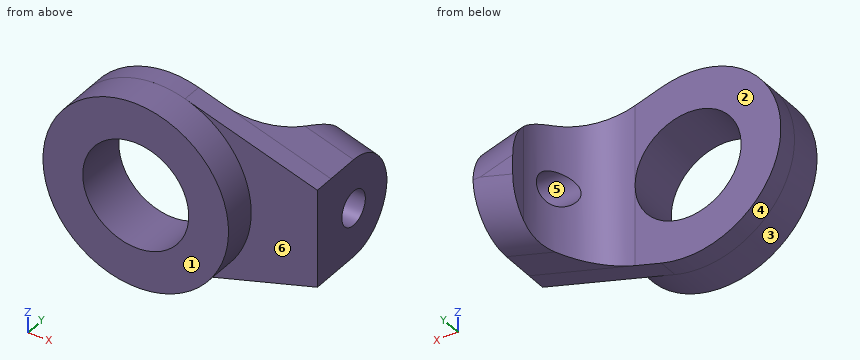
from build123d import *

# Parameters (mm, degrees)
SKETCH_1_R          = 7
EXTRUDE_1_DEPTH     = 1.5
SKETCH_3_R          = 4
CUT_EXTRUDE_2_DEPTH = 11.012492197
EXTRUDE_START       = -1.5
SKETCH_5_R          = 7
EXTRUDE_2_DEPTH     = 1.5
SKETCH_11_R         = 7
SKETCH_11_R_2       = 4
EXTRUDE_4_DEPTH     = 2.5
EXTRUDE_6_DEPTH     = 6.2
FILLET_1_R          = 5
SKETCH_12_R         = 1.3
CUT_EXTRUDE_3_DEPTH = 22.663858813
FILLET_2_R          = 3.7


with BuildPart() as part:
    # Эскиз1 → Бобышка-Вытянуть1 (new body)
    with BuildSketch(Plane(origin=(0, 0, 0), x_dir=(1, 0, 0), z_dir=(0, 1, 0))):
        with Locations(Location((0, 0, 0), (0, 0, 270))):
            Circle(SKETCH_1_R)
    extrude(amount=EXTRUDE_1_DEPTH)

    # Эскиз3 → Вырез-Вытянуть2 (cut, through all)
    with BuildSketch(Plane(origin=(0, 1.5, 0), x_dir=(1, 0, 0), z_dir=(0, 1, 0))):
        with Locations(Location((0, 0, 0), (0, 0, 270))):
            Circle(SKETCH_3_R)
    extrude(amount=-CUT_EXTRUDE_2_DEPTH, mode=Mode.SUBTRACT)

    # Эскиз5 → Бобышка-Вытянуть2 (add)
    with BuildSketch(Plane(origin=(0, 1.5, 0), x_dir=(1, 0, 0), z_dir=(0, 1, 0)).offset(EXTRUDE_START)):
        with BuildLine():
            ThreePointArc((2.017080382, 6.703746112), (-7.000630343, 0), (2.017080382, -6.703746112))
            Line((2.017080382, -6.703746112), (12, -3.7))
            Line((12, -3.7), (12, 3.7))
            Line((12, 3.7), (2.017080382, 6.703746112))
        make_face()
        Circle(SKETCH_5_R, mode=Mode.SUBTRACT)
    extrude(amount=EXTRUDE_2_DEPTH)

    # Эскиз11 → Бобышка-Вытянуть4 (add)
    with BuildSketch(Plane(origin=(0, 0, 0), x_dir=(-1, 0, 0), z_dir=(0, -1, 0))):
        with Locations(Location((0, 0, 0), (0, 0, 270))):
            Circle(SKETCH_11_R)
        with Locations(Location((0, 0, 0), (0, 0, 270))):
            Circle(SKETCH_11_R_2, mode=Mode.SUBTRACT)
    extrude(amount=EXTRUDE_4_DEPTH)

    # Эскиз13 → Бобышка-Вытянуть6 (add)
    with BuildSketch(Plane(origin=(0, 1.5, 0), x_dir=(1, 0, 0), z_dir=(0, 1, 0))):
        Polygon((9, 4.602665621), (9, 0), (9, -4.602665621), (12, -3.7), (12, 3.7), align=None)
    extrude(amount=EXTRUDE_6_DEPTH)

    # Скругление1
    fillet_1_edges = [part.edges().sort_by_distance(p)[0] for p in [
        (9, 1.5, 0),
    ]]
    fillet(fillet_1_edges, radius=FILLET_1_R)

    # Эскиз12 → Вырез-Вытянуть3 (cut, through all)
    with BuildSketch(Plane(origin=(12, 0, 0), x_dir=(0, 0, -1), z_dir=(1, 0, 0))):
        with Locations((0, 4)):
            Circle(SKETCH_12_R)
    extrude(amount=-CUT_EXTRUDE_3_DEPTH, mode=Mode.SUBTRACT)

    # Скругление2
    # the kernel refuses this fillet: 3.7 mm, written as the material it takes off along each edge
    with BuildSketch(Plane(origin=(0.142275982, 7.7, 7.267853272), x_dir=(0, -1, 0), z_dir=(0.9575917857777037, 0, -0.28812839466298473)), Plane(origin=(20.857724018, 7.7, -1.034812349), x_dir=(0, -1, 0), z_dir=(-0.9575917857777037, 0, -0.28812839466298473))) as fillet_2_piece_1:
        with BuildLine():
            CenterArc((FILLET_2_R, FILLET_2_R), FILLET_2_R, 180, 90)
            Line((0, FILLET_2_R), (0, 0))
            Line((0, 0), (FILLET_2_R, 0))
        make_face()
    extrude(amount=21.632858954, mode=Mode.SUBTRACT)


solid = part.part
Can you work these out from the model? Positions are in its coordinate system, mm. Face numbers are marked on the shaded views. A direction names the side the tool comes from. Coordinates: 2 decimals unless noted, no trailing zeros. Order: outer loops, then holes, each group sorted by start corner. A loop starts at its lowest first (then second) coordinate and runs counter-clockwise, first axis right, second up. Notation, with made-up numbers: (88, 86.5) - (140, 86.5) arc R21 cw to (140, 94.5) - close; hole circle Ø5 at (80, -27). An arc over 180 degrees is marked (long way). Answer as a JSON object with one key per item and string values. Group by question number.
Q1. We'd pull the mould along Z, two halves only. Please class the marked faces 4, 5 and 6: +Z half, -Z half, draft (parallel to the pull), parting line (faces both ways), or undercut.
Q2. On a 3-axis mill with a long thin cutter (end or side, diameter ignored), from which of +Z, -Z, +X, -X, +Y, -Y can I reach the whole of each face in a straight line? I mean the marked faces 1, 2 and 3. Say none if no direction works.
Q3. Imagine slicing it at C-C (y = 2.25). Please give me the cut outline in (x, z).
Q4. Will these pins go through, and if not, where does the flat tip stop? P1, Ø3, axis at y = 4, z = 0, coming from the -X side; P2, Ø1.5, axis at x = 7.5, y = 0, coming from the -Z side; P3, Ø1.3, axis at y = 7, z = -1, coming from the -X side.
Q5. Imagine slicing it at D-D (x = 6.25). Please give me the cut outline in (y, z).
Q6. I need wall thicknesses on line 1 (Y direction, x = 10.9, z = 0); line 2 (X direction, y = -0.65, z = 0); line 3 (Y direction, x = 8.75, z = 0). Which ranges of each line are inside material? Lowest first, please. Write a range as from..to.
Determined:
{
 "1": {"face 4": "parting line", "face 5": "undercut", "face 6": "draft"},
 "2": {"face 1": "+Z, -Z, +X, -X, -Y", "face 2": "+Z, -Z, -X, +Y", "face 3": "-Y"},
 "3": {"outline": "(6.63, -5.31) - (12, -3.7) - (12, 3.7) - (6.63, 5.31) - close"},
 "4": {"P1": "stops at x = 7", "P2": "stops at z = -5.28", "P3": "stops at x = 9"},
 "5": {"outline": "(-2.5, -3.15) - (0, -3.15) - (0, -5.43) - (2.03, -5.43) - (2.03, 5.43) - (0, 5.43) - (0, 3.15) - (-2.5, 3.15) - close"},
 "6": {"line 1": "y = 0..2.7, 5.3..7.7", "line 2": "x = -7..-4, 4..7", "line 3": "y = 0..2.7"}
}
